Could you check a few things on this model? Use its own coordinates, in mm. Face numbers are marked on the shaded views. A direction names the side the tool comes from. Round coordinates to 2 decimals unless told otherwise and drop trailing zeros. Write each loop counter-clockwise with the first axis right and the second up, starting at its lowest first coordinate (ties: lowest second). Pieces come first, ordered by that corner, then holes.
```python
from build123d import *

# Parameters (mm, degrees)
BOSS_EXTRUDE2_DEPTH = 159
SKETCH4_W           = 6
SKETCH4_H           = 151
CUT_EXTRUDE1_DEPTH  = 20


with BuildPart() as part:
    # Sketch3 → Boss-Extrude2 (new body)
    with BuildSketch(Plane.XY):
        Polygon((0, 0), (0, 105.870341046), (10, 105.870341046), (10, 23.872751767), (91.212923353, 23.872751767), (91.212923353, 105.870341046), (101.212923353, 105.870341046), (101.212923353, 0), align=None)
    extrude(amount=BOSS_EXTRUDE2_DEPTH)

    # Sketch4 → Cut-Extrude1 (cut)
    with BuildSketch(Plane(origin=(0, 105.870341046, 0), x_dir=(1, 0, 0), z_dir=(0, 1, 0))):
        with Locations((5, -79.5)):
            Rectangle(SKETCH4_W, SKETCH4_H)
        with Locations((96.212923353, -79.5)):
            Rectangle(SKETCH4_W, SKETCH4_H)
    extrude(amount=-CUT_EXTRUDE1_DEPTH, mode=Mode.SUBTRACT)


solid = part.part
```
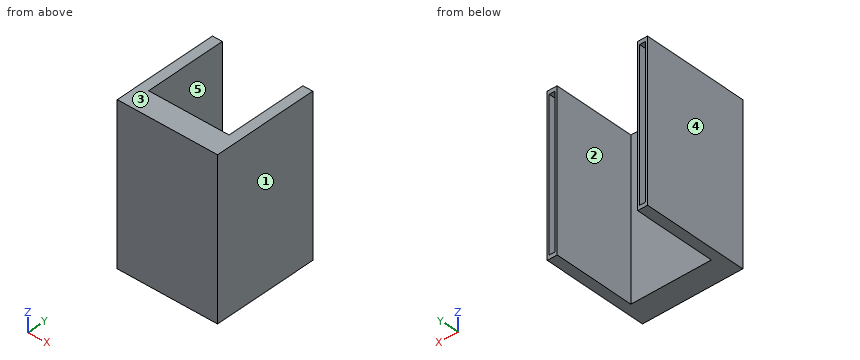
Q1. Imagine slicing it at B-B, the plane y = 70. Write out the boundary of the cut face in (x, z), then the cut area to 3 significant figures.
Q2. We'd pull the mould along X, two halves only. Please class the marked faces 3, 4 and 5: pulls with the +X half, pulls with the -X half, needs draft (parallel to the pull), parting line crosses it, or undercut.
Q3. Imagine slicing it at C-C, the plane z = 145. Write out the boundary of the cut face in (x, y), then the cut area to 3 significant figures.
Q4. If I drill on L1, parallel to X at y = 98, z = 99; L2, parallel to X at y = 65.5, z = 52; L3, parallel to Z at x = 5.5, y = 86.5, over which ranges is the centre line in solid material (lowest first)?
Q5. Imagine slicing it at A-A, the plane y = 93.5. Write out the boundary of the cut face in (x, z).
Q6. I'm going to push flat-ended pins straight in: pin 1 Ø5 at (x, z) = (97.5, 94) entering from +Y; pin 2 Ø8 at (x, y) = (85.5, 30) entering from -Z; pin 3 Ø10 at (x, z) = (81, 141.5) entering from +Y. Where does each tip first touch, or does it pass through?
Q7. On a 3-axis mill with a long thin cutter (end or side, diameter ignored), from which of +Z, -Z, +X, -X, +Y, -Y can I reach the whole of each face in a straight line? I mean the marked faces 1 and 2. Say none if no direction works.
Q8. Imagine slicing it at D-D, the plane x = 13. Write out the boundary of the cut face in (y, z), then the cut area to 3 significant figures.
Results found:
1. outline: (0, 0) - (10, 0) - (10, 159) - (0, 159) - close; (91.21, 0) - (101.21, 0) - (101.21, 159) - (91.21, 159) - close
1. area: 3,180 mm2
2. face 3: needs draft
2. face 4: pulls with the -X half
2. face 5: undercut
3. outline: (0, 0) - (101.21, 0) - (101.21, 105.87) - (99.21, 105.87) - (99.21, 85.87) - (93.21, 85.87) - (93.21, 105.87) - (91.21, 105.87) - (91.21, 23.87) - (10, 23.87) - (10, 105.87) - (8, 105.87) - (8, 85.87) - (2, 85.87) - (2, 105.87) - (0, 105.87) - close
3. area: 3,820 mm2
4. L1: x = 0 to 2, 8 to 10, 91.21 to 93.21, 99.21 to 101.21
4. L2: x = 0 to 10, 91.21 to 101.21
4. L3: z = 0 to 4, 155 to 159
5. outline: (0, 0) - (10, 0) - (10, 159) - (0, 159) - close; (91.21, 0) - (101.21, 0) - (101.21, 159) - (91.21, 159) - close; hole (2, 4) - (8, 4) - (8, 155) - (2, 155) - close; hole (93.21, 4) - (99.21, 4) - (99.21, 155) - (93.21, 155) - close
6. pin 1: stops at y = 105.87
6. pin 2: passes through
6. pin 3: stops at y = 23.87
7. face 1: +Z, -Z, +X, +Y, -Y
7. face 2: +Z, -Z, +Y
8. outline: (0, 0) - (23.87, 0) - (23.87, 159) - (0, 159) - close
8. area: 3,800 mm2
